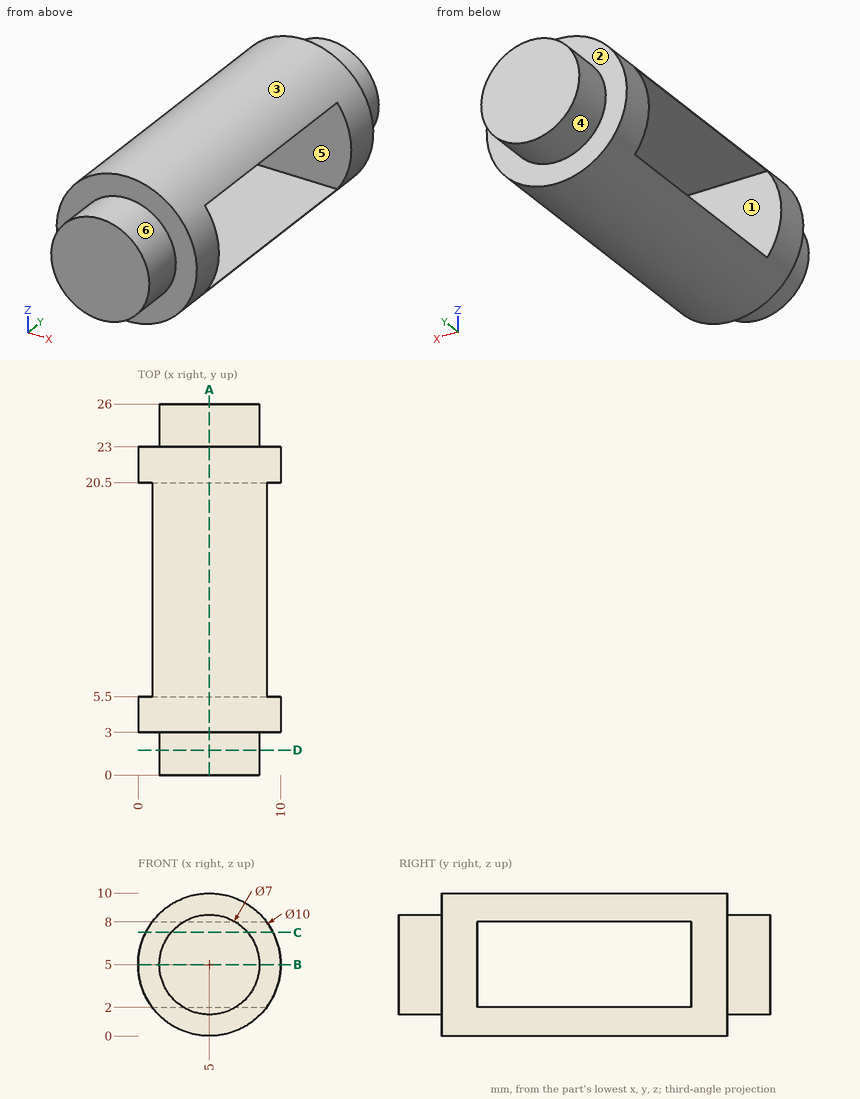
Geometry check sheet. Reference: drawing and pictorial views, mm from the part's lowest x, y, z. A direction names the side the tool comes from. Give positions to 0.01 mm unless a question says otherwise; leave off trailing zeros. Order: outer loops, then holes, each group sorted by start corner. A loop starts at its lowest first (then second) coordinate and runs counter-clockwise, first axis right, second up. Notation, with made-up numbers: M 62.5,30.25 L 84.5,30.25 A29 cw 84.5,68.25 Z; hole C -0.5,-4 d5. An arc over 180 degrees is marked long. Return JSON: item names as keys, results as strings. Group by question number.
1) Section check A-A on x = 5. Record the cut outline in (y, z).
2) Scan lines: line 1 (Y direction, x = 8.5, z = 4.25); line 2 (Y direction, x = 5, z = 7.25); line 3 (Z direction, x = 2, y = 9.75). Record each from-to range of solid material in increasing order.
3) Section check B-B on z = 5. Record the cut outline in (x, y), and give its area (3 significant figures).
4) Section check D-D on y = 1.75. Record the cut outline in (x, z), and give its area (3 significant figures).
5) Mould release check, pull along Z, two halves, no side actions. Record for the marked faces 1, 2 and 3: pulls with the +Z half, pulls with the -Z half, needs draft (parallel to the pull), parting line crosses it, or undercut.
6) Go/stop test with flat-tipped pins: pin 1 Ø1.5 at (y, z) = (21, 6.5) entering from -X; pin 2 Ø1.5 at (y, z) = (12.5, 2.5) entering from +X; pin 3 Ø6 at (x, z) = (6.5, 9) entering from +Y; pin 4 Ø1 at (x, y) = (8, 6.5) entering from +Z. Record where each tip stops, or that it passes through.
7) Access from +Z, -Z, +X, -X, +Y, -Y to the whole of each face (thin tool, end or side, straight path). Record for the marked faces 4, 5 and 6.
8) Section check C-C on z = 7.25. Record the cut outline in (x, y).
Answer block:
{
 "1": {"outline": "M 0,1.5 L 3,1.5 L 3,0 L 23,0 L 23,1.5 L 26,1.5 L 26,8.5 L 23,8.5 L 23,10 L 3,10 L 3,8.5 L 0,8.5 Z; hole M 5.5,2 L 20.5,2 L 20.5,8 L 5.5,8 Z"},
 "2": {"line 1": "y = 3 to 5.5, 20.5 to 23", "line 2": "y = 0 to 5.5, 20.5 to 26", "line 3": "z = 1 to 2, 8 to 9"},
 "3": {"outline": "M 0,3 L 1.5,3 L 1.5,0 L 8.5,0 L 8.5,3 L 10,3 L 10,5.5 L 0,5.5 Z; M 0,20.5 L 10,20.5 L 10,23 L 8.5,23 L 8.5,26 L 1.5,26 L 1.5,23 L 0,23 Z", "area": "92.0 mm^2"},
 "4": {"outline": "C 5,5 d7", "area": "38.5 mm^2"},
 "5": {"face 1": "undercut", "face 2": "needs draft", "face 3": "parting line crosses it"},
 "6": {"pin 1": "stops at x = 0.06", "pin 2": "stops at x = 9", "pin 3": "stops at y = 26", "pin 4": "stops at z = 9.33"},
 "7": {"face 4": "+Y", "face 5": "+X, -X", "face 6": "-Y"},
 "8": {"outline": "M 0.53,3 L 2.32,3 L 2.32,0 L 7.68,0 L 7.68,3 L 9.47,3 L 9.47,5.5 L 0.53,5.5 Z; M 0.53,20.5 L 9.47,20.5 L 9.47,23 L 7.68,23 L 7.68,26 L 2.32,26 L 2.32,23 L 0.53,23 Z"}
}
